The listing builds one solid part. Answer for the finished solid, in the listing's coordinates (mm). Face numbers are marked on the shaded views. Coordinates: 2 decimals unless noted, no trailing zeros. Order: outer loops, then holes, each group sorted by start corner. A loop starts at its lowest first (then second) coordinate and runs counter-clockwise, first axis right, second up. Notation, with made-up numbers: (-12.5, 61) -> (18.5, 61) arc R33 cw to (18.5, 99) -> close; hole circle Ø11 at (-19, -6). An arc over 180 degrees is marked (long way). Put each result on its own line as item: value. Start each with the question number.
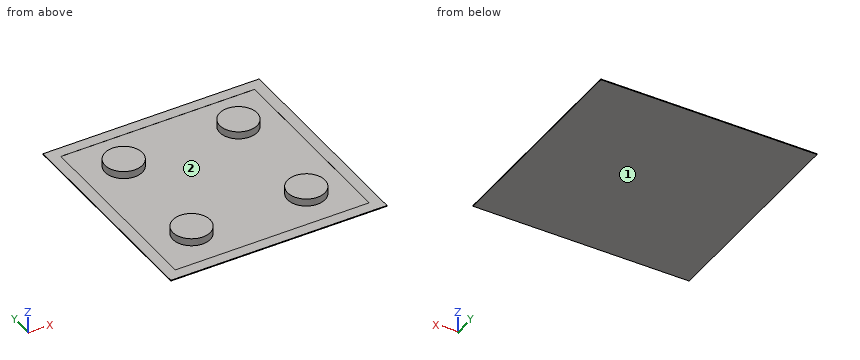
```python
from build123d import *

# Parameters (mm, degrees)
F0_W     = 73.66
F0_H     = 73.66
F1_DEPTH = 0.254
F2_W     = 73.66
F2_H     = 73.66
F2_W_2   = 66.04
F2_H_2   = 66.04
F3_DEPTH = 0.0254
F4_R     = 6.35
F5_DEPTH = 2.54


with BuildPart() as f1:
    # F0 (on Top) → F1 (new body)
    with BuildSketch(Plane.XY):
        with Locations((36.83, 36.83)):
            Rectangle(F0_W, F0_H)
    extrude(amount=F1_DEPTH)

    # F2 (on face) → F3 (join)
    with BuildSketch(Plane.XY.offset(0.254)):
        with Locations((36.83, 36.83)):
            Rectangle(F2_W, F2_H)
        with Locations((36.83, 36.83)):
            Rectangle(F2_W_2, F2_H_2, mode=Mode.SUBTRACT)
    extrude(amount=F3_DEPTH)

    # F4 (on face) → F5 (join)
    with BuildSketch(Plane.XY.offset(0.254)):
        with Locations((17.280384, 56.379616)):
            Circle(F4_R)
        with Locations((17.280384, 17.280384)):
            Circle(F4_R)
        with Locations((56.379616, 17.280384)):
            Circle(F4_R)
        with Locations((56.379616, 56.379616)):
            Circle(F4_R)
    extrude(amount=F5_DEPTH)


solid = f1.part
```
(1) The part is cut by section C-C on z = 2.05. Determine the outline of the cut face in (x, y), plus the area to 3 significant figures.
(2) Find the intervals of material crossed by L1, parallel to X at y = 56, z = 1.15; L2, parallel to Z at x = 37.5, y = 30; L3, parallel to Y at x = 62, z = 0.9, in increasing order.
(3) For a pull along Y with two mould halves and no side action, classify the marked faces 1 and 2 as released by +Y, released by -Y, zero draft, split by the parting line, or undercut.
(4) Each of these flat-tipped pins is pushed along its axis until it touches: P1, Ø1.5, axis at y = 14, z = 1.5, coming from the +X side; P2, Ø3, axis at x = 9.5, y = 15.5, coming from the -Z side; P3, Ø1.5, axis at x = 19.5, y = 48, coming from the +Z side; P4, Ø1.5, axis at x = 19, z = 2, coming from the -Y side. Where does it stop, or does it pass through?
Worked out:
1. outline: circle Ø12.7 at (17.28, 17.28); circle Ø12.7 at (17.28, 56.38); circle Ø12.7 at (56.38, 17.28); circle Ø12.7 at (56.38, 56.38)
1. area: 507 mm2
2. L1: 10.94 to 23.62, 50.04 to 62.72
2. L2: 0 to 0.25
2. L3: 14.33 to 20.24, 53.42 to 59.33
3. face 1: zero draft
3. face 2: undercut
4. P1: x = 62.2
4. P2: z = 0
4. P3: z = 0.25
4. P4: y = 11
